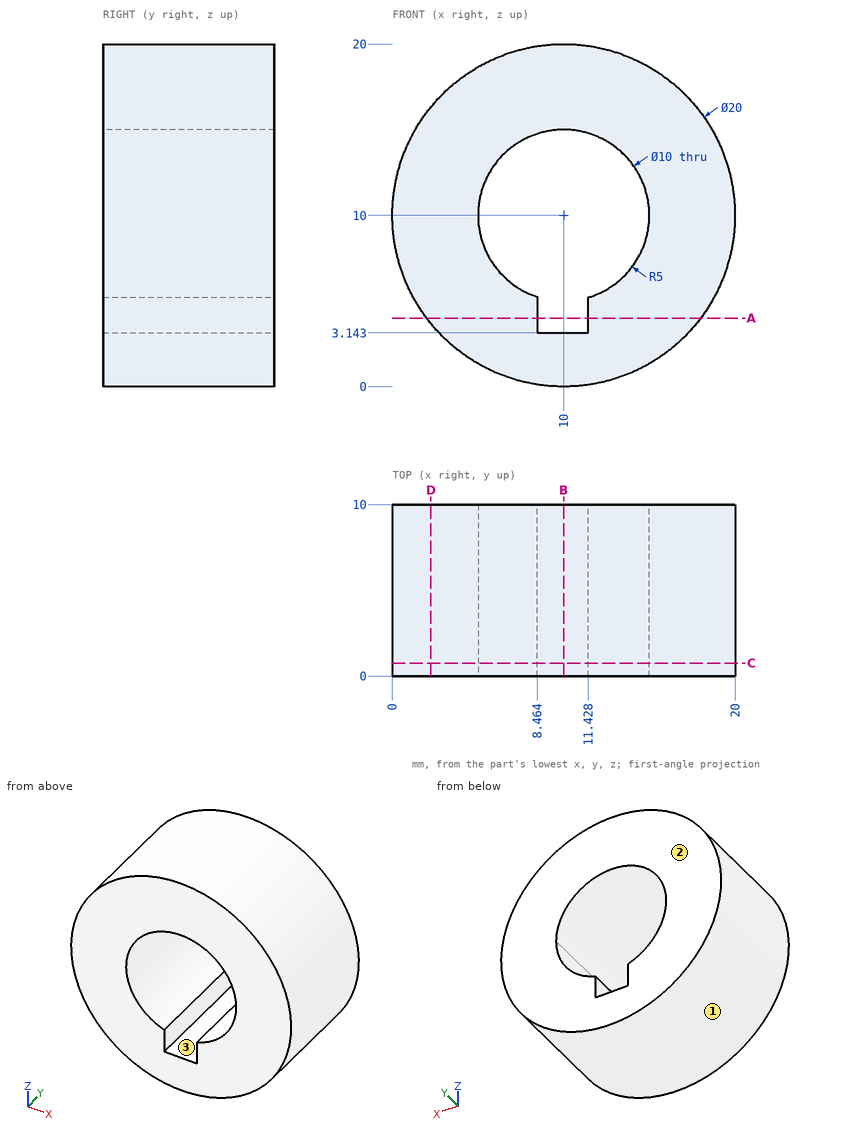
Check sheet for the drawn part. Datum: minimum x, y, z corner. Units: mm. Give positions to 0.01 mm unless a question says otherwise; leave off trailing zeros. Loops run counter-clockwise (first coordinate to the right, second up) from the corner with the lowest first, then second, coordinate; pieces in that order, holes last. Notation, with made-up numbers: M 31.25,62.25 L 69.25,62.25 A24 cw 69.25,72.25 Z; hole C 29,25 d3. An arc over 180 degrees is marked long. Return JSON: item names as keys, results as strings.
1) Section check B-B, the plane x = 10. Enter the section's corners in (y, z).
Findings:
{"outline": "M 0,0 L 10,0 L 10,3.14 L 0,3.14 Z; M 0,15 L 10,15 L 10,20 L 0,20 Z"}
2) Mould release check, pull along Z, two halves, no side actions. Record for the marked faces 1, 2 and 3: released by +Z, released by -Z, zero draft, split by the parting line, or undercut.
Findings:
{"face 1": "split by the parting line", "face 2": "zero draft", "face 3": "undercut"}
3) Section check A-A, the plane z = 4. Enter the section's corners in (x, y), and give its area (3 significant figures).
Findings:
{"outline": "M 2,0 L 8.46,0 L 8.46,10 L 2,10 Z; M 11.43,0 L 18,0 L 18,10 L 11.43,10 Z", "area": "130 mm2"}
4) Section check D-D, the plane x = 2.25. Enter the section's corners in (y, z), and give its area (3 significant figures).
Findings:
{"outline": "M 0,3.68 L 10,3.68 L 10,16.32 L 0,16.32 Z", "area": "126 mm2"}
5) Section check C-C, the plane y = 0.75. Enter the section's corners in (x, z), and give its area (3 significant figures).
Findings:
{"outline": "C 10,10 d20; hole M 8.46,3.14 L 11.43,3.14 L 11.43,5.21 A5 ccw long 8.46,5.24 Z", "area": "230 mm2"}
6) Gauge pin test, flat ends, axial feed: P1, Ø1, axis at y = 5.5, z = 16.5, coming from the +X side; P2, Ø1.5, axis at x = 4.5, y = 8, coming from the +Z side; P3, Ø3, axis at x = 7.5, y = 2.5, coming from the -Z side; P4, Ø4, axis at x = 8, z = 11, coming from the +Y side. Record the tip position at first contact, or that the pin passes through.
Findings:
{"P1": "stops at x = 18", "P2": "stops at z = 18.8", "P3": "stops at z = 0.05", "P4": "passes through"}
7) Material ranges on L1, parallel to X at y = 5, z = 10; L2, parallel to X at y = 7.75, z = 14.5, recorded low to high. Write a range as [from, to].
Findings:
{"L1": "x = [0, 5], [15, 20]", "L2": "x = [1.07, 7.82], [12.18, 18.93]"}
